```python
from build123d import *

# Parameters (mm, degrees)
SKETCH1_W           = 49.5
SKETCH1_H           = 50.000619057
BOSS_EXTRUDE1_DEPTH = 10
CUT_EXTRUDE1_DEPTH  = 8
SKETCH4_R           = 1.45
CUT_EXTRUDE2_DEPTH  = 8
SKETCH5_R           = 2.75
CUT_EXTRUDE3_DEPTH  = 1
SKETCH6_R           = 5
CUT_EXTRUDE4_DEPTH  = 3


with BuildPart() as part:
    # Sketch1 → Boss-Extrude1 (new body)
    with BuildSketch(Plane.XY):
        with Locations((1.875288206, 25.000309529)):
            Rectangle(SKETCH1_W, SKETCH1_H)
    extrude(amount=BOSS_EXTRUDE1_DEPTH)

    # Sketch3 → Cut-Extrude1 (cut)
    with BuildSketch(Plane(origin=(0, 0, 0), x_dir=(-1, 0, 0), z_dir=(0, 0, -1))):
        with BuildLine():
            Line((17.871256182, -0.2), (14.760723675, 5.183428821))
            ThreePointArc((14.760723675, 5.183428821), (10.522339102, 13.396152422), (6.2841063, 5.183350498))
            Line((6.2841063, 5.183350498), (4.25724424, 1.67))
            Line((4.25724424, 1.67), (-8.010847692, 1.67))
            Line((-8.010847692, 1.67), (-10.03930416, 5.183389663))
            ThreePointArc((-10.03930416, 5.183389663), (-14.277636876, 13.396152423), (-18.5158937, 5.183350498))
            Line((-18.5158937, 5.183350498), (-21.621564167, -0.2))
            Line((-21.621564167, -0.2), (17.871256182, -0.2))
        make_face()
    extrude(amount=-CUT_EXTRUDE1_DEPTH, mode=Mode.SUBTRACT)

    # Sketch4 → Cut-Extrude2 (cut)
    with BuildSketch(Plane(origin=(0, 0, 8), x_dir=(-1, 0, 0), z_dir=(0, 0, -1))):
        with Locations((-14.27761285, 8.196152423)):
            Circle(SKETCH4_R)
        with Locations((10.52238715, 8.196152423)):
            Circle(SKETCH4_R)
    extrude(amount=-CUT_EXTRUDE2_DEPTH, mode=Mode.SUBTRACT)

    # Sketch5 → Cut-Extrude3 (cut)
    with BuildSketch(Plane.XY.offset(10)):
        with Locations((-10.52238715, 8.196152423)):
            Circle(SKETCH5_R)
        with Locations((14.27761285, 8.196152423)):
            Circle(SKETCH5_R)
    extrude(amount=-CUT_EXTRUDE3_DEPTH, mode=Mode.SUBTRACT)

    # Sketch6 → Cut-Extrude4 (cut)
    with BuildSketch(Plane(origin=(0, 0, 0), x_dir=(-1, 0, 0), z_dir=(0, 0, -1))):
        with Locations((-1.875273442, 33.500619057)):
            Circle(SKETCH6_R)
    extrude(amount=-CUT_EXTRUDE4_DEPTH, mode=Mode.SUBTRACT)


solid = part.part
```
Check sheet for the modelled part. Datum: model origin and axes. Units: mm. A direction names the side the tool comes from. Coordinates: 2 decimals unless noted, no trailing zeros. Write each loop counter-clockwise with the first axis right and the second up, starting at its lowest first coordinate (ties: lowest second). Pieces come first, ordered by that corner, then holes. Notation, with made-up numbers: M 86.5,60.25 L 139.5,60.25 A18 ccw 139.5,75.25 Z; hole C 83.25,2 d9. An arc over 180 degrees is marked long. Use one line per item in the form item = value.
Item 1: Sectioned sample at C-C, the plane z = 4.75. Record the cut outline in (x, y).
Answer below:
outline = M -22.87,0 L -17.76,0 L -14.76,5.18 A5.2 cw long -6.28,5.18 L -4.26,1.67 L 8.01,1.67 L 10.04,5.18 A5.2 cw long 18.52,5.18 L 21.51,0 L 26.63,0 L 26.63,50 L -22.87,50 Z
Item 2: Sectioned sample at B-B, the plane x = 15. Record the cut outline in (y, z).
Answer below:
outline = M 0,8 L 6.94,8 L 6.94,9 L 5.54,9 L 5.54,10 L 0,10 Z; M 9.45,8 L 13.35,8 L 13.35,0 L 50,0 L 50,10 L 10.85,10 L 10.85,9 L 9.45,9 Z
Item 3: Gauge pin test, flat ends, axial feed: pin 1 Ø4.5 at (x, y) = (-10.52, 8.2) entering from +Z; pin 2 Ø5 at (x, z) = (-3, 4.5) entering from -Y; pin 3 Ø4.5 at (x, y) = (14.28, 8.2) entering from -Z. Record the tip position at first contact, or that the pin passes through.
Answer below:
pin_1 = 9
pin_2 = 1.67
pin_3 = 8
Item 4: Release check for a two-part mould opening along Y. For faces 1 (the face through (-12.549, 10.055, 9.507)), 2 (the face through (-22.875, 25, 5)), 3 (the face through (2, 50.001, 5)), 4 (the face through (1.5, 0, 8.3)) record: pulls with the +Y half, pulls with the -Y half, needs draft (parallel to the pull), parting line crosses it, or undercut.
Answer below:
face_1 = undercut
face_2 = needs draft
face_3 = pulls with the +Y half
face_4 = pulls with the -Y half
Item 5: Sectioned sample at D-D, the plane z = 2. Record the cut outline in (x, y).
Answer below:
outline = M -22.87,0 L -17.76,0 L -14.76,5.18 A5.2 cw long -6.28,5.18 L -4.26,1.67 L 8.01,1.67 L 10.04,5.18 A5.2 cw long 18.52,5.18 L 21.51,0 L 26.63,0 L 26.63,50 L -22.87,50 Z; hole C 1.88,33.5 d10
Item 6: Sectioned sample at A-A, the plane y = 9. Record the cut outline in (x, z).
Answer below:
outline = M -22.87,0 L -15.66,0 L -15.66,8 L -11.73,8 L -11.73,9 L -13.15,9 L -13.15,10 L -22.87,10 Z; M -9.32,8 L -5.38,8 L -5.38,0 L 9.14,0 L 9.14,8 L 13.07,8 L 13.07,9 L 11.65,9 L 11.65,10 L -7.89,10 L -7.89,9 L -9.32,9 Z; M 15.48,8 L 19.42,8 L 19.42,0 L 26.63,0 L 26.63,10 L 16.91,10 L 16.91,9 L 15.48,9 Z
Item 7: Set-up check for faces 5 (the face through (-16.279, 2.555, 3.944)), 6 (the face through (15.5, 7, 9)), 7 (the face through (26.625, 25, 5)), 8 (the face through (-9.372, 7.314, 8.493)), 9 (the face through (2, 34, 3)): record each of +Z, -Z, +X, -X, +Y, -Y from which the full face is reachable in a straight line by a thin tool's end or side.
Answer below:
face_5 = -Z, -Y
face_6 = +Z
face_7 = +Z, -Z, +X, +Y, -Y
face_8 = +Z, -Z
face_9 = -Z
Item 8: Material ranges on L1, parallel to X at y = 8, z = 2.5; L2, parallel to Z at x = 12, y = 7.5; L3, parallel to Y at x = -10.5, z = 4, recorded low to high. Write a range as from..to.
Answer below:
L1 = -22.87..-15.72, -5.33..9.08, 19.47..26.63
L2 = 8..9
L3 = 13.4..50
